Model file for the job. Use its own axes, mm. Face numbers are marked on the shaded views. A direction names the side the tool comes from. Round coordinates to 2 decimals unless told otherwise and drop trailing zeros. Loops run counter-clockwise (first coordinate to the right, second up) from the corner with the lowest first, then second, coordinate; pieces in that order, holes last. Notation, with made-up numbers: M 34.5,67 L 38.5,67 A20 cw 38.5,102 Z; hole C 26,88.5 d4. An arc over 180 degrees is marked long. Use a Markdown table: item, result. Add a question column.
Q1. Mould opens along Z. For the marked faces 1, 2, 3 and 4 say: +Z half, -Z half, draft (parallel to the pull), parting line (faces both ways), or undercut.
Q2. Cut at C-C (z = 23.5). Give the cut face in (x, y).
Q3. Tool access for the marked faces 5, 6 and 7: list every direction of +Z, -Z, +X, -X, +Y, -Y with a clear straight run to the whole face (end or side of a thin tool).
Q4. Cut at A-A (y = -52). State how many separate pieces and enclosed holes the cut face has, plus the area to 3 significant figures.
Q5. Probe line 1 (Z direction, x = -49, y = -47.5); line 2 (Z direction, x = 55.5, y = -12); line 3 (X direction, y = -14.5, z = 12). List the from-to ranges inside material, lowest first. Write a range as from..to.
Q6. Cut at B-B (x = 17). Give the cut face in (y, z).
Q7. Pin check, flat tips, straight feed: pin 1 (1.5 mm diameter, centred on x = 8.5, z = 17.5, fed in from -Y); pin 2 (1 mm diameter, centred on x = 54.5, z = 14, fed in from +Y); pin 3 (1.5 mm diameter, centred on x = -58.5, z = 45, fed in from +Y). Stop position of each tip, or through.
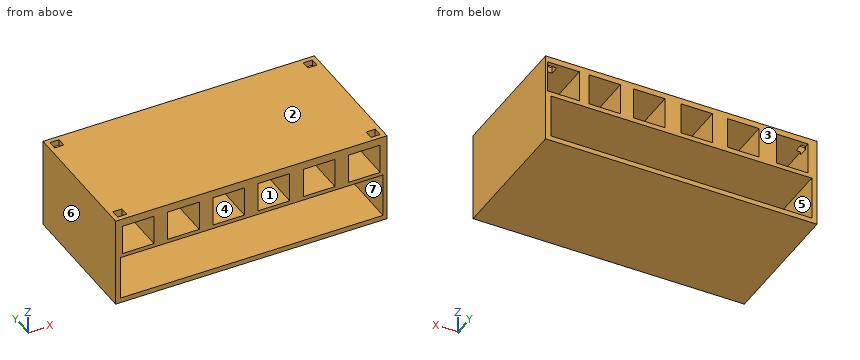
from build123d import *

# Parameters (mm, degrees)
F0_W      = 152.4
F0_H      = 25.4
F1_DEPTH  = 76.2
F2_W      = 17.78
F2_H      = 17.78
F2_H_2    = 17.502186
F2_H_3    = 17.781453
F3_DEPTH  = 33.02
F4_W      = 17.78
F4_H      = 16.6878
F5_DEPTH  = 33.02
F6_W      = 146.541581
F6_H      = 24.47215
F7_DEPTH  = 33.02
F8_W      = 147.48656
F8_H      = 24.775412
F10_DEPTH = 33.02
F11_W     = 5.08
F11_H     = 5.08
F11_H_2   = 4.8768
F11_H_3   = 5.080004
F12_DEPTH = 5.08


with BuildPart() as f1:
    # F0 (on Front) → F1 (new body)
    with BuildSketch(Plane.XZ):
        with Locations((-6.284538, 38.1)):
            Rectangle(F0_W, F0_H)
        with Locations((-6.284538, 12.7)):
            Rectangle(F0_W, F0_H)
    extrude(amount=F1_DEPTH)

    # F2 (on Front) → F3 (cut)
    with BuildSketch(Plane.XZ):
        with Locations((-68.533134, 38.567891)):
            Rectangle(F2_W, F2_H)
        with Locations((-41.029694, 38.706798)):
            Rectangle(F2_W, F2_H_2)
        with Locations((-14.915321, 38.673893)):
            Rectangle(F2_W, F2_H_3)
        with Locations((11.754678, 38.673893)):
            Rectangle(F2_W, F2_H_3)
        with Locations((36.757799, 38.673893)):
            Rectangle(F2_W, F2_H_3)
        with Locations((59.816236, 38.673893)):
            Rectangle(F2_W, F2_H_3)
    extrude(amount=F3_DEPTH, mode=Mode.SUBTRACT)

    # F4 (on face) → F5 (cut)
    with BuildSketch(Plane.XZ.offset(76.2)):
        with Locations((-69.784538, 38.026275)):
            Rectangle(F4_W, F4_H)
        with Locations((-44.384538, 38.026275)):
            Rectangle(F4_W, F4_H)
        with Locations((-18.984538, 38.026275)):
            Rectangle(F4_W, F4_H)
        with Locations((6.415462, 38.026275)):
            Rectangle(F4_W, F4_H)
        with Locations((31.815462, 38.026275)):
            Rectangle(F4_W, F4_H)
        with Locations((57.215462, 38.026275)):
            Rectangle(F4_W, F4_H)
    extrude(amount=-F5_DEPTH, mode=Mode.SUBTRACT)

    # F6 (on Front) → F7 (cut)
    with BuildSketch(Plane.XZ):
        with Locations((-6.280116, 14.999481)):
            Rectangle(F6_W, F6_H)
    extrude(amount=F7_DEPTH, mode=Mode.SUBTRACT)

    # F8 (on face) → F10 (cut)
    with BuildSketch(Plane.XZ.offset(76.2)):
        with Locations((-6.05702, 15.156722)):
            Rectangle(F8_W, F8_H)
    extrude(amount=-F10_DEPTH, mode=Mode.SUBTRACT)

    # F11 (on face) → F12 (cut)
    with BuildSketch(Plane.XY.offset(50.8)):
        with Locations((-77.404538, -5.08)):
            Rectangle(F11_W, F11_H)
        with Locations((64.835462, -4.9784)):
            Rectangle(F11_W, F11_H_2)
        with Locations((64.835462, -71.12)):
            Rectangle(F11_W, F11_H)
        with Locations((-77.404538, -71.119998)):
            Rectangle(F11_W, F11_H_3)
    extrude(amount=-F12_DEPTH, mode=Mode.SUBTRACT)


solid = f1.part
Checked values:
| question | item | result |
|---|---|---|
| 1 | face 1 | undercut |
| 1 | face 2 | +Z half |
| 1 | face 3 | draft |
| 1 | face 4 | undercut |
| 2 | outline | M -82.48,-76.2 L -79.8,-76.2 L -79.8,-43.18 L 67.69,-43.18 L 67.69,-76.2 L 69.92,-76.2 L 69.92,0 L 66.99,0 L 66.99,-33.02 L -79.55,-33.02 L -79.55,0 L -82.48,0 Z |
| 3 | face 5 | +Y |
| 3 | face 6 | +Z, -Z, -X, +Y, -Y |
| 3 | face 7 | -Y |
| 4 | separate pieces | 1 |
| 4 | enclosed holes | 7 |
| 4 | area | 2,310 mm^2 |
| 5 | line 1 | z = 0..2.77, 27.54..29.68, 46.37..50.8 |
| 5 | line 2 | z = 0..2.76, 27.24..29.78, 47.56..50.8 |
| 5 | line 3 | x = -82.48..-79.55, 66.99..69.92 |
| 6 | outline | M -76.2,0 L 0,0 L 0,2.76 L -33.02,2.76 L -33.02,27.24 L 0,27.24 L 0,29.78 L -33.02,29.78 L -33.02,47.56 L 0,47.56 L 0,50.8 L -76.2,50.8 L -76.2,27.54 L -43.18,27.54 L -43.18,2.77 L -76.2,2.77 Z |
| 7 | pin 1 | stops at y = -43.18 |
| 7 | pin 2 | stops at y = -33.02 |
| 7 | pin 3 | stops at y = 0 |
